from build123d import *

# Parameters (mm, degrees)
SKETCH1_R           = 12.75
BOSS_EXTRUDE1_DEPTH = 8
SKETCH2_W           = 2
SKETCH2_H           = 0.4
BOSS_EXTRUDE2_DEPTH = 0.2
SKETCH3_W           = 2
SKETCH3_H           = 0.4
BOSS_EXTRUDE3_DEPTH = 0.2
SKETCH4_W           = 2
SKETCH4_H           = 0.4
BOSS_EXTRUDE4_DEPTH = 0.2
CHAMFER1_SIZE       = 0.2
SKETCH5_W           = 2
SKETCH5_H           = 0.4
BOSS_EXTRUDE5_DEPTH = 0.2
CHAMFER2_SIZE       = 0.2


with BuildPart() as part:
    # Sketch1 → Boss-Extrude1 (new body)
    with BuildSketch(Plane(origin=(0, 0, 0), x_dir=(1, 0, 0), z_dir=(0, 1, 0))):
        with Locations(Location((0, 0, 0), (0, 0, 270))):
            Circle(SKETCH1_R)
        with BuildLine():
            Line((-1, 10.703387314), (1, 10.703387314))
            ThreePointArc((1, 10.703387314), (7.601397898, 7.601397898), (10.703387314, 1))
            Line((10.703387314, 1), (10.703387314, -1))
            ThreePointArc((10.703387314, -1), (7.601397898, -7.601397898), (1, -10.703387314))
            Line((1, -10.703387314), (-1, -10.703387314))
            ThreePointArc((-1, -10.703387314), (-7.601397898, -7.601397898), (-10.703387314, -1))
            Line((-10.703387314, -1), (-10.703387314, 1))
            ThreePointArc((-10.703387314, 1), (-7.601397898, 7.601397898), (-1, 10.703387314))
        make_face(mode=Mode.SUBTRACT)
    extrude(amount=BOSS_EXTRUDE1_DEPTH)

    # Sketch2 → Boss-Extrude2 (add)
    with BuildSketch(Plane.XY.offset(-10.703387314)):
        with Locations((0, 0.2)):
            Rectangle(SKETCH2_W, SKETCH2_H)
    extrude(amount=BOSS_EXTRUDE2_DEPTH)

    # Sketch3 → Boss-Extrude3 (add)
    with BuildSketch(Plane(origin=(-10.703387314, 0, 0), x_dir=(0, 0, -1), z_dir=(1, 0, 0))):
        with Locations((0, 0.2)):
            Rectangle(SKETCH3_W, SKETCH3_H)
    extrude(amount=BOSS_EXTRUDE3_DEPTH)

    # Sketch4 → Boss-Extrude4 (add)
    with BuildSketch(Plane(origin=(0, 0, 10.703387314), x_dir=(-1, 0, 0), z_dir=(0, 0, -1))):
        with Locations((0, 0.2)):
            Rectangle(SKETCH4_W, SKETCH4_H)
    extrude(amount=BOSS_EXTRUDE4_DEPTH)

    # Chamfer1
    chamfer1_edges = [part.edges().sort_by_distance(p)[0] for p in [
        (1, 0.2, -10.503387314),
        (-1, 0.2, -10.503387314),
        (-10.503387314, 0.2, 1),
        (-10.503387314, 0.2, -1),
        (-1, 0.2, 10.503387314),
        (1, 0.2, 10.503387314),
    ]]
    chamfer(chamfer1_edges, length=CHAMFER1_SIZE - 0.0001)  # a hair under: the kernel refuses the full size

    # Sketch5 → Boss-Extrude5 (add)
    with BuildSketch(Plane.ZY.offset(-10.703387314)):
        with Locations((0, 0.2)):
            Rectangle(SKETCH5_W, SKETCH5_H)
    extrude(amount=BOSS_EXTRUDE5_DEPTH)

    # Chamfer2
    chamfer2_edges = [part.edges().sort_by_distance(p)[0] for p in [
        (10.503387314, 0.2, 1),
        (10.503387314, 0.2, -1),
    ]]
    chamfer(chamfer2_edges, length=CHAMFER2_SIZE - 0.0001)  # a hair under: the kernel refuses the full size


solid = part.part
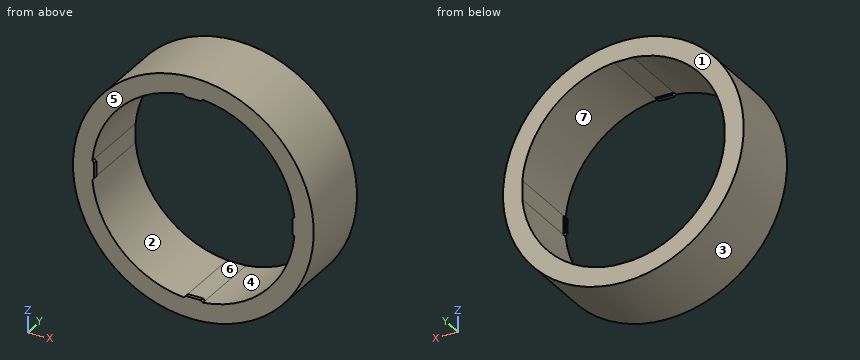
Input: part model. Units: mm. Frame: model coordinates. Face numbers are marked on the shaded views. A direction names the side the tool comes from. Coordinates: 2 decimals unless noted, no trailing zeros. Loops run counter-clockwise (first coordinate to the right, second up) from the corner with the lowest first, then second, coordinate; pieces in that order, holes last. Notation, with made-up numbers: (-6, 82) -> (38, 82) arc R15 ccw to (38, 94) -> close; hole circle Ø11 at (34, 49.5). An arc over 180 degrees is marked (long way). Write item = value, one per line. Start each with the question number.
Item 1: Cut plane C-C, the plane x = 0. Return loops of the section in (y, z), plus the area to 3 significant figures.
Item 2: Material intervals for line 1 (X direction, y = 7.75, z = -9.25); line 2 (Z direction, x = -8.5, y = 5); line 3 (Z direction, x = -7.75, y = 0.5), sorted ascending.
Item 3: Mould query, pull axis X, two halves, no side actions, for the marked faces 1, 2, 3 and 4. Classes: pulls with the +X half, pulls with the -X half, needs draft (parallel to the pull), parting line crosses it, or undercut.
Item 4: Cut plane B-B, the plane y = 7.5. Return loops of the section in (x, z).
Item 5: Cut plane A-A, the plane z = 0. Return loops of the section in (x, y).
Item 6: Cut plane D-D, the plane z = -5. Return loops of the section in (x, y).
Item 7: Reachability of the marked faces 5, 6 and 7 from +Z, -Z, +X, -X, +Y, -Y: full face, straight path, thin tool, end or side. Return the list, or none.
Item 8: First-contact query: P1, Ø4, axis at y = 7, z = -6, coming from the -X side. Flat tip, straight axial feed; report the tip coordinate or a pass-through.
Ans:
q1.outline = (0, -12.75) -> (8, -12.75) -> (8, -10.7) -> (0.4, -10.7) -> (0.4, -10.5) -> (0, -10.5) -> close; (0, 10.5) -> (0.4, 10.5) -> (0.4, 10.7) -> (8, 10.7) -> (8, 12.75) -> (0, 12.75) -> close
q1.area = 32.9 mm²
q2.line_1 = -8.77 to -5.48, 5.48 to 8.77
q2.line_2 = -9.5 to -6.58, 6.58 to 9.5
q2.line_3 = -10.12 to -7.45, 7.45 to 10.12
q3.face_1 = needs draft
q3.face_2 = undercut
q3.face_3 = parting line crosses it
q3.face_4 = undercut
q4.outline = circle Ø25.5 at (0, 0); hole (-10.7, -1) arc R10.75 ccw to (-1, -10.7) -> (1, -10.7) arc R10.75 ccw to (10.7, -1) -> (10.7, 1) arc R10.75 ccw to (1, 10.7) -> (-1, 10.7) arc R10.75 ccw to (-10.7, 1) -> close
q5.outline = (-12.75, 0) -> (-10.5, 0) -> (-10.5, 0.4) -> (-10.7, 0.4) -> (-10.7, 8) -> (-12.75, 8) -> close; (10.5, 0) -> (12.75, 0) -> (12.75, 8) -> (10.7, 8) -> (10.7, 0.4) -> (10.5, 0.4) -> close
q6.outline = (-11.73, 0) -> (-9.52, 0) -> (-9.52, 8) -> (-11.73, 8) -> close; (9.52, 0) -> (11.73, 0) -> (11.73, 8) -> (9.52, 8) -> close
q7.face_5 = +Z, -Z, +X, -X, -Y
q7.face_6 = +Y
q7.face_7 = +Y, -Y
q8.P1 = -12.11
